```python
from build123d import *

# Parameters (mm, degrees)
F0_W     = 2.0066
F0_H     = 12.4968
F0_W_2   = 19.05
F0_H_2   = 12.7
F0_H_3   = 1.27
F1_DEPTH = 3.175


# Not quite as in the source:
# - a length typed as a fraction of an inch, garbled in the dataset ("3 / 203.2 mm" for 3/8 in), is restored


with BuildPart() as f1:
    # F0 (on Top) → F1 (new body)
    with BuildSketch(Plane.XY):
        Polygon((-63.5, 0), (0, 0), (0, 127), (-63.5, 127), (-63.5, 13.97), (-44.45, 13.97), (-44.45, 12.7), (-63.5, 12.7), align=None)
        with Locations((-24.1173, 54.3814)):
            Rectangle(F0_W, F0_H, mode=Mode.SUBTRACT)
        Polygon((-95.25, 0), (-82.55, 0), (-82.55, 12.7), (-82.55, 13.97), (-63.5, 13.97), (-63.5, 127), (-127, 127), (-127, 54.3814), (-127, 0), align=None)
        Polygon((-103.886, 48.133), (-103.886, 54.3814), (-103.886, 60.6298), (-101.8794, 60.6298), (-101.8794, 48.133), align=None, mode=Mode.SUBTRACT)
        with Locations((-73.025, 6.35)):
            Rectangle(F0_W_2, F0_H_2)
        with Locations((-73.025, 13.335)):
            Rectangle(F0_W_2, F0_H_3)
        with Locations((-53.975, 13.335)):
            Rectangle(F0_W_2, F0_H_3)
    extrude(amount=F1_DEPTH)


solid = f1.part
```
Verification items for the finished model (mm, model axes). A direction names the side the tool comes from. Give positions to 0.01 mm unless a question says otherwise; leave off trailing zeros. Order: outer loops, then holes, each group sorted by start corner. A loop starts at its lowest first (then second) coordinate and runs counter-clockwise, first axis right, second up. Notation, with made-up numbers: M 6.5,50.5 L 40.5,50.5 A10 ccw 40.5,67.5 Z; hole C 69.25,-25 d1. An arc over 180 degrees is marked long. Answer in a Markdown table with one row per item. Add a question column.
Item 1: Mould release check, pull along Y, two halves, no side actions. Record for faces 1 (the flat face through (-64, 64, 0)), 2 (the flat face through (-103.886, 54, 2)), 3 (the flat face through (-63, 127, 2)): released by +Y, released by -Y, zero draft, split by the parting line, or undercut.
Item 2: Section check A-A, the plane y = 53. Enter the section's corners in (x, z) (3 decimals).
Item 3: Tool access check on faces 4 (the flat face through (-23.114, 54, 2)), 5 (the flat face through (-64, 0, 2)). Record the directions out of +Z, -Z, +X, -X, +Y, -Y that give a thin tool (end or side, any length) a straight path to the whole face; none if there is none.
Item 4: Gauge pin test, flat end, axial feed: pin 1 (6 mm diameter, centred on x = -40.5, y = 84.5, fed in from -Z). Record the tip position at first contact, or that the pin passes through.
Filled sheet:
| question | item | result |
|---|---|---|
| 1 | face 1 | zero draft |
| 1 | face 2 | undercut |
| 1 | face 3 | released by +Y |
| 2 | outline | M -127,0 L -103.886,0 L -103.886,3.175 L -127,3.175 Z; M -101.879,0 L -25.121,0 L -25.121,3.175 L -101.879,3.175 Z; M -23.114,0 L 0,0 L 0,3.175 L -23.114,3.175 Z |
| 3 | face 4 | +Z, -Z |
| 3 | face 5 | +Z, -Z, +X, -X, -Y |
| 4 | pin 1 | stops at z = 0 |
